Design review of the part built by this model. Coordinates are the model's own, in mm. A direction names the side the tool comes from. Coordinates: 2 decimals unless noted, no trailing zeros. Loops run counter-clockwise (first coordinate to the right, second up) from the corner with the lowest first, then second, coordinate; pieces in that order, holes last. Notation, with made-up numbers: (-14, 2) -> (-2, 2) arc R21 cw to (-2, 28) -> close; hole circle Ø5 at (33.25, 17). An arc over 180 degrees is marked (long way). Answer in a Markdown table with one row per item.
```python
from build123d import *

# Parameters (mm, degrees)
F1_DEPTH = 55
F2_T     = -1
F4_DEPTH = 1


with BuildPart() as f1:
    # F0 (on Front) → F1 (new body, symmetric)
    with BuildSketch(Plane.XZ):
        with BuildLine():
            ThreePointArc((-181.3245903513, -365.2919652377), (-178.0253293171, -371.5628290115), (-171.3991288349, -374.0732718036))
            Line((-171.3991288349, -374.0732718036), (210.2621403614, -374.0732718036))
            ThreePointArc((210.2621403614, -374.0732718036), (216.8883408435, -371.5628290115), (220.1876018778, -365.2919652377))
            Line((220.1876018778, -365.2919652377), (292.6582958135, 224.9344720505))
            ThreePointArc((292.6582958135, 224.9344720505), (289.3590347792, 233.6427226924), (280.3136153411, 235.8561227473))
            Line((280.3136153411, 235.8561227473), (-230.6466922573, 108.4594097216))
            ThreePointArc((-230.6466922573, 108.4594097216), (-236.4687351875, 104.4205148281), (-238.1529348177, 97.5377590248))
            Line((-238.1529348177, 97.5377590248), (-181.3245903513, -365.2919652377))
        make_face()
    extrude(amount=F1_DEPTH, both=True)

    # F2 (hollow: no face is removed)
    offset(amount=F2_T, mode=Mode.SUBTRACT)

    # F3 (on face) → F4 (cut, through all)
    with BuildSketch(Plane(origin=(-38.9581795543, 0, 156.2527237618), x_dir=(0.9702957263, 0, 0.2419218956), z_dir=(-0.2419218956, 0, 0.9702957263))):
        with BuildLine():
            ThreePointArc((-7.1386698707, 25.4085332208), (-10.2738331899, 21.8343178236), (-11.404046427, 17.2162140156))
            Line((-11.404046427, 17.2162140156), (-11.404046427, -7.3706747529))
            ThreePointArc((-11.404046427, -7.3706747529), (-10.2738331899, -11.988778561), (-7.1386698707, -15.5629939581))
            Line((-7.1386698707, -15.5629939581), (11.0135524375, -28.2695495739))
            ThreePointArc((11.0135524375, -28.2695495739), (13.7417820324, -29.6146092552), (16.7481758812, -30.0772303687))
            Line((16.7481758812, -30.0772303687), (135.4437312648, -30.0772303687))
            ThreePointArc((135.4437312648, -30.0772303687), (138.4501251136, -29.6146092552), (141.1783547084, -28.2695495739))
            Line((141.1783547084, -28.2695495739), (159.3305770166, -15.5629939581))
            ThreePointArc((159.3305770166, -15.5629939581), (162.4657403358, -11.988778561), (163.595953573, -7.3706747529))
            Line((163.595953573, -7.3706747529), (163.595953573, 17.2162140156))
            ThreePointArc((163.595953573, 17.2162140156), (162.4657403358, 21.8343178236), (159.3305770166, 25.4085332208))
            Line((159.3305770166, 25.4085332208), (141.1783547084, 38.1150888365))
            ThreePointArc((141.1783547084, 38.1150888365), (138.4501251136, 39.4601485179), (135.4437312648, 39.9227696313))
            Line((135.4437312648, 39.9227696313), (16.7481758812, 39.9227696313))
            ThreePointArc((16.7481758812, 39.9227696313), (13.7417820324, 39.4601485179), (11.0135524375, 38.1150888365))
            Line((11.0135524375, 38.1150888365), (-7.1386698707, 25.4085332208))
        make_face()
    extrude(amount=-F4_DEPTH, mode=Mode.SUBTRACT)


solid = f1.part
```
(1) Take a section at C-C on z = -220. Give the boundary of the cut face in (x, y), and give its area (3 significant figures).
Evaluation:
| item | result |
|---|---|
| outline | (-199.16, -55) -> (238.03, -55) -> (238.03, 55) -> (-199.16, 55) -> close; hole (-198.16, -54) -> (237.02, -54) -> (237.02, 54) -> (-198.16, 54) -> close |
| area | 1,090 mm² |
(2) Tool access review of faces 5 (the flat face through (17, -1, -373.073)), 6 (the flat face through (34, -30.077, 174)), 7 (the flat face through (-37.08, -21.83, 156.21)), 8 (the flat face through (106.829, -22.005, 192.093)): name each direction out of +Z, -Z, +X, -X, +Y, -Y from which nothing blocks a thin tool from reaching the whole face with its end or side.
Evaluation:
| item | result |
|---|---|
| face 5 | none |
| face 6 | +Z, -X |
| face 7 | +Z |
| face 8 | -X |
(3) Take a section at B-B on x = -158. Give the boundary of the cut face in (y, z), and give its area (3 significant figures).
Evaluation:
| item | result |
|---|---|
| outline | (-55, -374.07) -> (55, -374.07) -> (55, 126.57) -> (-55, 126.57) -> close; hole (-54, -373.07) -> (54, -373.07) -> (54, 125.54) -> (-54, 125.54) -> close |
| area | 1,220 mm² |
(4) Take a section at D-D on x = 67. Give the boundary of the cut face in (y, z), and give its area (3 significant figures).
Evaluation:
| item | result |
|---|---|
| outline | (-55, -374.07) -> (55, -374.07) -> (55, 182.67) -> (39.92, 182.67) -> (39.92, 181.64) -> (54, 181.64) -> (54, -373.07) -> (-54, -373.07) -> (-54, 181.64) -> (-30.08, 181.64) -> (-30.08, 182.67) -> (-55, 182.67) -> close |
| area | 1,260 mm² |
(5) Draft analysis for pull direction X (two halves, no side actions). For faces 1 (the flat face through (24, 55, -65)), 2 (the flat face through (107.08, 31.67, 192.15)), 3 (the flat face through (24, 54, -65)), 4 (the flat face through (-209.144, -0.756, -130.515)), state which applies: pulls with the +X half, pulls with the -X half, needs draft (parallel to the pull), parting line crosses it, or undercut.
Evaluation:
| item | result |
|---|---|
| face 1 | needs draft |
| face 2 | pulls with the -X half |
| face 3 | undercut |
| face 4 | undercut |
(6) For pin 1 (1 mm diameter, centred on y = 17, z = -246.5, fed in from +X); pin 2 (4 mm diameter, centred on y = 10, z = -190, fed in from -X); pin 3 (6 mm diameter, centred on y = 16.5, z = -236, fed in from -X), all flat-tipped, find the tip position at first contact; note any pin that passes through.
Evaluation:
| item | result |
|---|---|
| pin 1 | stops at x = 234.83 |
| pin 2 | stops at x = -203.09 |
| pin 3 | stops at x = -197.57 |
(7) To check wall thickness, follow probe 1 along Y at (x, z) = (-103, 48); probe 2 along X at (y, z) = (24, -178); probe 3 along Z at (x, y) = (158, 32). State the ranges of each line that lie inside material, in increasing order.
Evaluation:
| item | result |
|---|---|
| probe 1 | y = -55 to -54, 54 to 55 |
| probe 2 | x = -204.32 to -203.31, 242.18 to 243.18 |
| probe 3 | z = -374.07 to -373.07, 204.33 to 205.36 |
(8) Take a section at A-A on y = -44. Give the boundary of the cut face in (x, z).
Evaluation:
| item | result |
|---|---|
| outline | (-238.15, 97.54) -> (-181.32, -365.29) arc R10 ccw to (-171.4, -374.07) -> (210.26, -374.07) arc R10 ccw to (220.19, -365.29) -> (292.66, 224.93) arc R10 ccw to (280.31, 235.86) -> (-230.65, 108.46) arc R10 ccw to start; hole (-237.16, 97.66) -> (-180.33, -365.17) arc R9 ccw to (-171.4, -373.07) -> (210.26, -373.07) arc R9 ccw to (219.2, -365.17) -> (291.67, 225.06) arc R9 ccw to (280.56, 234.89) -> (-230.4, 107.49) arc R9 ccw to start |
